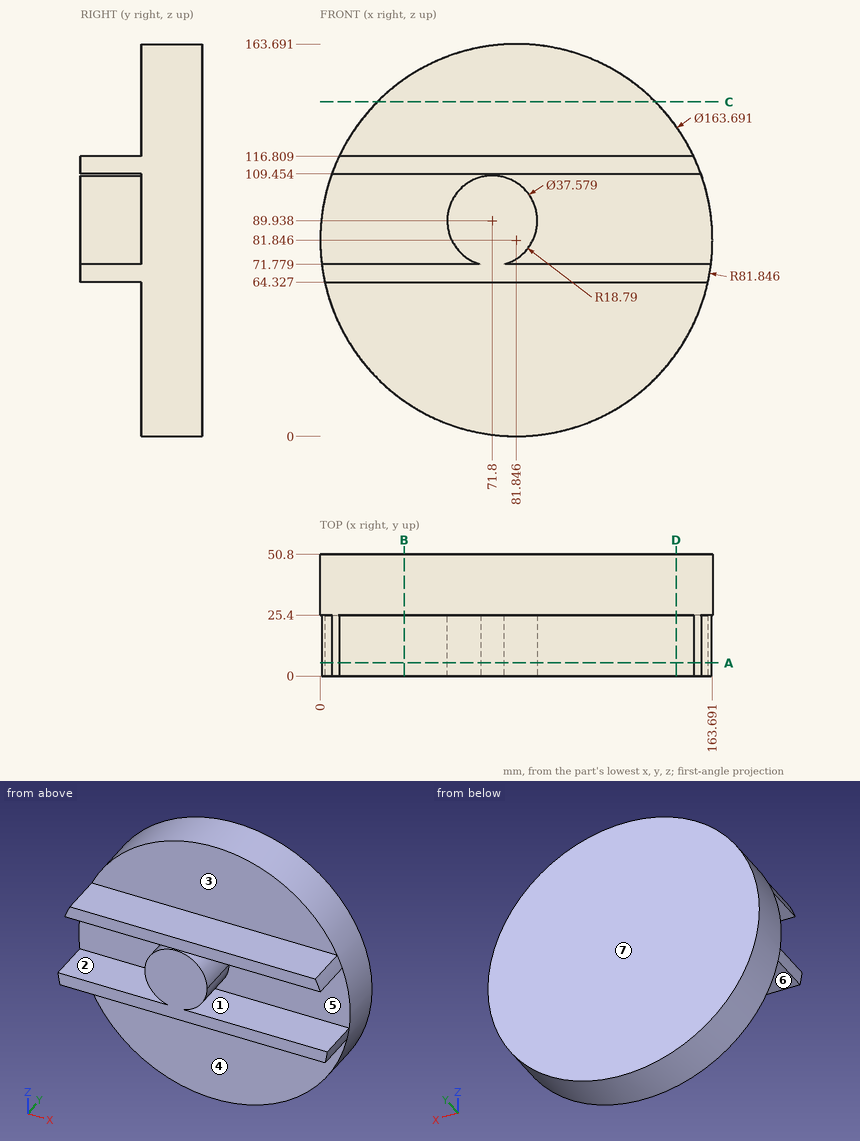
Job drawing, mm, ordinate dimensions from the low corner. One solid piece. A direction names the side the tool comes from. Give positions to 0.01 mm unless a question says otherwise; leave off trailing zeros. Loops run counter-clockwise (first coordinate to the right, second up) from the corner with the lowest first, then second, coordinate; pieces in that order, holes last. Notation, with made-up numbers: (-12.5, 48) -> (33.5, 48) arc R14 cw to (33.5, 52) -> close; hole circle Ø6 at (-26.75, 36.5). An arc over 180 degrees is marked (long way). Use a Markdown table: item, result. Add a question column.
(1) Slice it at D-D on x = 148.5. List the corners of the cut face in (y, z), and give its area (3 significant figures).
(2) Slice it at C-C on z = 139.5. List the corners of the cut face in (x, y), and give its area (3 significant figures).
(3) Slice it at A-A on y = 5.5. List the corners of the cut face in (x, z) (1 decimal), and give its area (3 significant figures).
(4) Drop flat-ended pins along their axis: pin 1 Ø7.5 at (x, y) = (67, 11.5) entering from -Z; pin 2 Ø3 at (y, z) = (37.5, 92) entering from -X; pin 3 Ø3 at (y, z) = (15, 61) entering from -X; pin 4 Ø8 at (x, y) = (96, 38.5) entering from +Z. Give the stop position or say it passes through.
(5) Tool access for the marked faces 1, 2, 3 and 4: list every direction of +Z, -Z, +X, -X, +Y, -Y with a clear straight run to the whole face (end or side of a thin tool).
(6) Mould opens along Z. For the marked faces 5, 6 and 7 say: +Z half, -Z half, draft (parallel to the pull), parting line (faces both ways), or undercut.
(7) Slice it at B-B on x = 35. List the corners of the cut face in (y, z), and give its area (3 significant figures).
(8) Wall check: line 1 along Z through (x, y) = (120, 24.5); line 2 along Y through (x, z) = (77.5, 24); line 3 along Z through (x, y) = (51, 32) (1 decimal). Give the ranges that are in metal, low to high.
Filled sheet:
| question | item | result |
|---|---|---|
| 1 | outline | (0, 64.33) -> (25.4, 64.33) -> (25.4, 34.35) -> (50.8, 34.35) -> (50.8, 129.34) -> (25.4, 129.34) -> (25.4, 116.81) -> (0, 116.81) -> (0, 109.45) -> (25.4, 109.45) -> (25.4, 71.78) -> (0, 71.78) -> close |
| 1 | area | 2,790 mm2 |
| 2 | outline | (23.75, 25.4) -> (139.94, 25.4) -> (139.94, 50.8) -> (23.75, 50.8) -> close |
| 2 | area | 2,950 mm2 |
| 3 | outline | (0.6, 71.8) arc R81.8 ccw to (1.9, 64.3) -> (161.8, 64.3) arc R81.8 ccw to (163.1, 71.8) -> (76.6, 71.8) arc R18.8 ccw (long way) to (67, 71.8) -> close; (4.8, 109.5) -> (158.9, 109.5) arc R81.8 ccw to (155.8, 116.8) -> (7.8, 116.8) arc R81.8 ccw to start |
| 3 | area | 3,420 mm2 |
| 4 | pin 1 | z = 64.33 |
| 4 | pin 2 | x = 0.46 |
| 4 | pin 3 | through |
| 4 | pin 4 | z = 163.06 |
| 5 | face 1 | +X, -Y |
| 5 | face 2 | -X, -Y |
| 5 | face 3 | +Z, +X, -X, -Y |
| 5 | face 4 | -Z, +X, -X, -Y |
| 6 | face 5 | undercut |
| 6 | face 6 | -Z half |
| 6 | face 7 | draft |
| 7 | outline | (0, 64.33) -> (25.4, 64.33) -> (25.4, 14.73) -> (50.8, 14.73) -> (50.8, 148.96) -> (25.4, 148.96) -> (25.4, 116.81) -> (0, 116.81) -> (0, 109.45) -> (25.4, 109.45) -> (25.4, 71.78) -> (0, 71.78) -> close |
| 7 | area | 3,790 mm2 |
| 8 | line 1 | 64.33 to 71.78, 109.45 to 116.81 |
| 8 | line 2 | 25.4 to 50.8 |
| 8 | line 3 | 6 to 157.7 |
